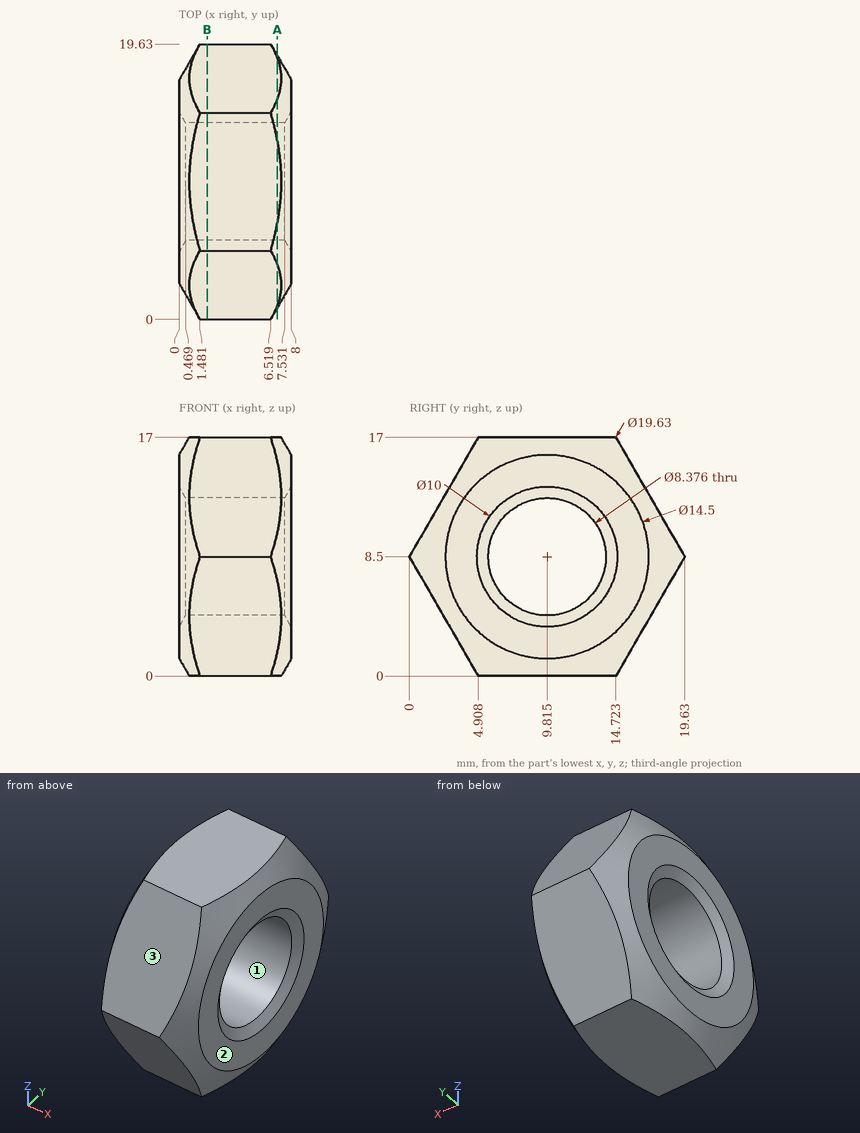
Study the drawing (mm; zero at the part's minimum x, y, z) and answer. Round coordinates to 2 decimals unless told otherwise and drop trailing zeros. Write each loop counter-clockwise with the first axis right and the second up, starting at its lowest first coordinate (ties: lowest second). Pieces come first, ordered by that corner, then holes. Notation, with made-up numbers: (-9, -9.75) -> (24, -9.75) arc R12 cw to (24, 12.25) -> close; hole circle Ø1 at (-20.5, 27.5). An arc over 180 degrees is marked (long way). Use CSV: the item, a comma, the result in double quotes. Start each with the question number.
(1) The mould has two halves that part along Y. Classify the marked faces 1, 2 and 3: released by +Y, released by -Y, zero draft, split by the parting line, or undercut.
(2) Section A-A on x = 7 is taken. Give the vertices of the cut face in (y, z) (1 decimal).
(3) Each of these flat-tipped pins is pushed along its axis until it touches: pin 1 (6 mm diameter, centred on y = 16, z = 4.5, fed in from +X); pin 2 (7.5 mm diameter, centred on y = 9.815, z = 8.5, fed in from -X); pin 3 (4 mm diameter, centred on x = 2.5, y = 17, fed in from +Z). Where does it stop, or does it pass through?
(4) Consider L1, parallel to Z at x = 1.75, y = 7; L2, parallel to Z at x = 4.25, y = 6 (1 decimal); L3, parallel to Z at x = 5, y = 3.5 (1 decimal). Determine where each line is inside the solid, lowest interval first. Write a range as from..to.
(5) Section B-B on x = 2 is taken. Give the vertices of the cut face in (y, z) (1 decimal).
A:
1,face 1,"undercut"
1,face 2,"zero draft"
1,face 3,"released by -Y"
2,outline,"(1, 6.8) -> (3.9, 1.7) arc R9 ccw to (6.9, 0) -> (12.7, 0) arc R9 ccw to (15.7, 1.7) -> (18.6, 6.8) arc R9 ccw to (18.6, 10.2) -> (15.7, 15.3) arc R9 ccw to (12.7, 17) -> (6.9, 17) arc R9 ccw to (3.9, 15.3) -> (1, 10.2) arc R9 ccw to start; hole circle Ø8.4 at (9.8, 8.5)"
3,pin 1,"stops at x = 8"
3,pin 2,"passes through"
3,pin 3,"stops at z = 16.52"
4,L1,"z = 0..5.4, 11.6..17"
4,L2,"z = 0..6.8, 10.2..17"
4,L3,"z = 2.4..14.6"
5,outline,"(0, 8.5) -> (4.9, 0) -> (14.7, 0) -> (19.6, 8.5) -> (14.7, 17) -> (4.9, 17) -> close; hole circle Ø8.4 at (9.8, 8.5)"
